Verification items for the finished model (mm, model axes). Round coordinates to 2 decimals unless told otherwise and drop trailing zeros. Write each loop counter-clockwise with the first axis right and the second up, starting at its lowest first coordinate (ties: lowest second). Pieces come first, ordered by that corner, then holes. Notation, with made-up numbers: M 0.5,68.25 L 8.5,68.25 A27 ccw 8.5,91.25 Z; hole C 10,17.5 d7. An arc over 180 degrees is marked long. Write each question's results on one line, items separated by ' | '.
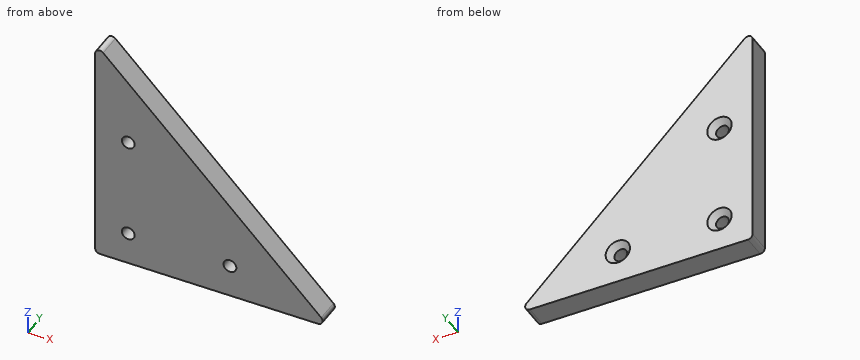
from build123d import *

# Parameters (mm, degrees)
BOSS_EXTRUDE1_DEPTH                             = 10
CSK_FOR_M5_FLAT_HEAD_MACHINE_SCREW1_D           = 5.5
CSK_FOR_M5_FLAT_HEAD_MACHINE_SCREW1_CSINK_D     = 10.4
CSK_FOR_M5_FLAT_HEAD_MACHINE_SCREW1_CSINK_ANGLE = 90
FILLET2_R                                       = 2


with BuildPart() as part:
    # Sketch1 → Boss-Extrude1 (new body)
    with BuildSketch(Plane(origin=(0, 0, 0), x_dir=(1, 0, 0), z_dir=(0, 1, 0))):
        Polygon((0, 0), (0, -100), (100, 0), align=None)
    extrude(amount=BOSS_EXTRUDE1_DEPTH)

    # CSK for M5 Flat Head Machine Screw1 (through all)
    with Locations(Plane(origin=(14.142135624, 10, 14.142135624), x_dir=(0, 0, 1), z_dir=(0, 1, 0))):
        with Locations((0, 0), (43.431457505, 0), (0, 43.431457505)):
            CounterSinkHole(CSK_FOR_M5_FLAT_HEAD_MACHINE_SCREW1_D / 2, CSK_FOR_M5_FLAT_HEAD_MACHINE_SCREW1_CSINK_D / 2, counter_sink_angle=CSK_FOR_M5_FLAT_HEAD_MACHINE_SCREW1_CSINK_ANGLE)

    # Fillet2
    fillet2_edges = [part.edges().sort_by_distance(p)[0] for p in [
        (100, 5, 0),
        (0, 5, 100),
        (0, 5, 0),
    ]]
    fillet(fillet2_edges, radius=FILLET2_R)


solid = part.part
1) Depth check by flat-ended pin: P1, Ø4, axis at x = 62.5, y = 5, coming from the +Z side; P2, Ø5, axis at x = 19, y = 3.5, coming from the +Z side; P3, Ø5, axis at x = 31.5, y = 3, coming from the +Z side. Enter the tip coordinate at first touch or a pass-through.
Calculated:
P1: stops at z = 39.5 | P2: stops at z = 83.5 | P3: stops at z = 71
2) Sectioned sample at A-A, the plane y = 4.5. Record the cut outline in (x, z), and give its area (3 significant figures).
Calculated:
outline: M 0,2 A2 ccw 2,0 L 95.17,0 A2 ccw 96.59,3.41 L 3.41,96.59 A2 ccw 0,95.17 Z; hole C 14.14,14.14 d5.5; hole C 14.14,57.57 d5.5; hole C 57.57,14.14 d5.5 | area: 4,920 mm²
3) Sectioned sample at C-C, the plane x = 38.5. Record the cut outline in (y, z).
Calculated:
outline: M 0,0 L 10,0 L 10,61.5 L 0,61.5 Z
4) Sectioned sample at B-B, the plane z = 67.5. Record the cut outline in (x, y).
Calculated:
outline: M 0,0 L 32.5,0 L 32.5,10 L 0,10 Z
5) Material ranges on line 1 (X direction, y = 5.5, z = 15.5); line 2 (Z direction, x = 57.5, y = 9.5); line 3 (X direction, y = 3, z = 56.5), recorded low to high. Write a range as [from, to].
Calculated:
line 1: x = [0, 11.75], [16.53, 55.18], [59.96, 84.5] | line 2: z = [0, 9.44], [18.84, 42.5] | line 3: x = [0, 11.61], [16.67, 43.5]
